Read the model definition and answer for the solid it produces. Units are mm, in the model's axes. A direction names the side the tool comes from. Coordinates: 2 decimals unless noted, no trailing zeros. Loops run counter-clockwise (first coordinate to the right, second up) from the corner with the lowest first, then second, coordinate; pieces in that order, holes last. Notation, with made-up numbers: (30, -16.75) -> (57, -16.75) arc R10 ccw to (57, -7.75) -> close; hole circle Ø8 at (-35, 60). An arc over 180 degrees is marked (long way). Answer as a JSON object with one key per item and string values. Group by question number.
1) Section B-B, the plane y = 22 is taken. Give the vertices of the cut face in (x, z), plus the area to 3 significant figures.
2) Flat-ended cylindrical pins translate along their axes: P1, Ø6.5, axis at x = 5, z = 0, coming from the -Y side; P2, Ø6, axis at y = 21.5, z = -7.5, coming from the -X side; P3, Ø1, axis at x = 9, y = 17, coming from the +Z side. Find the tip coordinate at first contact, or state that the pin passes through.
3) Determine the mould class of faces 4 (the face through (0.1, 12.4, 8.5)), 5 (the face through (10.74, 21.48, 2.38)), 6 (the face through (-8, 9.2, 2.4)) for opening direction X: released by +X, released by -X, zero draft, split by the parting line, or undercut.
4) Consider probe 1 along X at (y, z) = (17.5, -0.25); probe 2 along X at (y, z) = (4.75, 0); probe 3 along Y at (x, z) = (-2.25, 3). Determine where each line is inside the solid, lowest interval first. Write a range as [from, to].
5) Which of the six approach directions +Z, -Z, +X, -X, +Y, -Y give full straight-line access (tool end or side, diameter ignored) to faces 1 (the face through (10, 0, 1)), 2 (the face through (5, 14, 2)), 3 (the face through (10, 17, -1))?
from build123d import *

# Parameters (mm, degrees)
CUT_EXTRUDE1_DEPTH      = 19
CUT_EXTRUDE2_DEPTH      = 32.160872902
CUT_EXTRUDE2_DEPTH_BACK = 32.160872902
SKETCH3_R               = 3


with BuildPart() as part:
    # Sketch1 → Revolve1 (revolve)
    with BuildSketch(Plane.XY, mode=Mode.PRIVATE) as revolve1_sk:
        with BuildLine():
            Line((0, 27), (-6.5, 27))
            Line((-6.5, 27), (-11, 23))
            Line((-11, 23), (-11, 20))
            Line((-11, 20), (-9.75, 20))
            Line((-9.75, 20), (-9.75, 19))
            Line((-9.75, 19), (-11, 19))
            Line((-11, 19), (-11, 18))
            Line((-11, 18), (-9.75, 18))
            Line((-9.75, 18), (-9.75, 17))
            Line((-9.75, 17), (-11, 17))
            Line((-11, 17), (-11, 14))
            ThreePointArc((-11, 14), (-10.250666035, 11), (-11, 8))
            Line((-11, 8), (-11, 0))
            Line((-11, 0), (-9.75, 0))
            Line((-9.75, 0), (-9.75, 6))
            Line((-9.75, 6), (0, 6))
            Line((0, 6), (0, 27))
        make_face()
    revolve(revolve1_sk.sketch.rotate(Axis((0, -30.957446809, 0), (0, 1, 0)), 270), axis=Axis((0, -30.957446809, 0), (0, 1, 0)))

    # Sketch2 → Cut-Extrude1 (cut)
    with BuildSketch(Plane(origin=(0, 0, 0), x_dir=(1, 0, 0), z_dir=(0, 1, 0))):
        with BuildLine():
            Line((-5, -3.5), (-5, 3.5))
            ThreePointArc((-5, 3.5), (0, 8.5), (5, 3.5))
            Line((5, 3.5), (5, -3.5))
            ThreePointArc((5, -3.5), (0, -8.5), (-5, -3.5))
        make_face()
    extrude(amount=CUT_EXTRUDE1_DEPTH, mode=Mode.SUBTRACT)

    # Sketch3 → Cut-Extrude2 (cut, two sides: drawn at the far end of the back side and taken through both)
    with BuildSketch(Plane(origin=(0, 0, 0), x_dir=(0, 0, -1), z_dir=(1, 0, 0)).offset(-CUT_EXTRUDE2_DEPTH_BACK)):
        with Locations((0, 11)):
            Circle(SKETCH3_R)
    extrude(amount=CUT_EXTRUDE2_DEPTH + CUT_EXTRUDE2_DEPTH_BACK, mode=Mode.SUBTRACT)


solid = part.part
Determined:
{
 "1": {"outline": "circle Ø22 at (0, 0)", "area": "380 mm²"},
 "2": {"P1": "y = 6", "P2": "x = -10.04", "P3": "z = 6.98"},
 "3": {"face 4": "undercut", "face 5": "split by the parting line", "face 6": "zero draft"},
 "4": {"probe 1": "[-9.75, -5], [5, 9.75]", "probe 2": "[-11, -9.75], [9.75, 11]", "probe 3": "[19, 27]"},
 "5": {"face 1": "+Z, -Z, +X, -X, -Y", "face 2": "-Y", "face 3": "none"}
}
